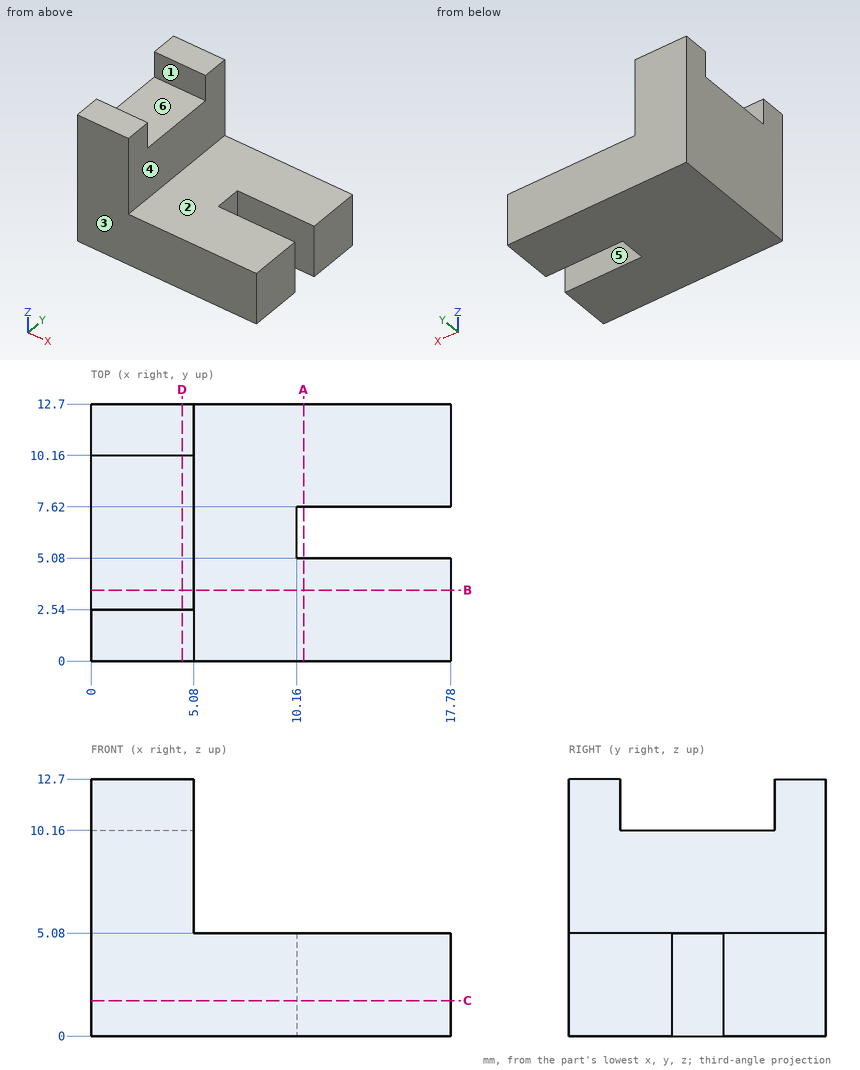
Answer from the drawing. Dimensions are ordinates in mm from the lowest x, y and z of the part. A direction names the side the tool comes from. Coordinates: 2 decimals unless noted, no trailing zeros. Loops run counter-clockwise (first coordinate to the right, second up) from the corner with the lowest first, then second, coordinate; pieces in that order, holes last. Notation, with made-up numbers: (61.25, -38.5) -> (118.25, -38.5) arc R20 ccw to (118.25, -3.5) -> close; hole circle Ø11 at (20.5, 38.25). An arc over 180 degrees is marked (long way). Return JSON: item names as keys, results as strings.
Item 1: Find section D-D (x = 4.5). Determine the outline of the cut face in (y, z), plus the area to 3 significant figures.
Answers:
{"outline": "(0, 0) -> (12.7, 0) -> (12.7, 12.7) -> (10.16, 12.7) -> (10.16, 10.16) -> (2.54, 10.16) -> (2.54, 12.7) -> (0, 12.7) -> close", "area": "142 mm2"}
Item 2: For a pull along Y with two mould halves and no side action, classify the marked faces 1, 2 and 3 as +Y half, -Y half, draft (parallel to the pull), parting line (faces both ways), or undercut.
Answers:
{"face 1": "undercut", "face 2": "draft", "face 3": "-Y half"}
Item 3: Find the intervals of material crossed by probe 1 along Y at (x, z) = (11.5, 1.5); probe 2 along X at (y, z) = (2.25, 12.25); probe 3 along Z at (x, y) = (1, 7.75), in increasing order.
Answers:
{"probe 1": "y = 0 to 5.08, 7.62 to 12.7", "probe 2": "x = 0 to 5.08", "probe 3": "z = 0 to 10.16"}
Item 4: Flat-ended cylindrical pins translate along their axes: P1, Ø2, axis at y = 9.5, z = 9.5, coming from the +X side; P2, Ø2, axis at x = 15.5, y = 7.5, coming from the -Z side; P3, Ø1.3, axis at y = 6.5, z = 1.5, coming from the +X side; P4, Ø1.5, axis at x = 15, y = 2.5, coming from the +Z side. Find the tip coordinate at first contact, or state that the pin passes through.
Answers:
{"P1": "stops at x = 5.08", "P2": "stops at z = 0", "P3": "stops at x = 10.16", "P4": "stops at z = 5.08"}
Item 5: For the marked faces 4, 5 and 6, determine the directions among +Z, -Z, +X, -X, +Y, -Y from which every point of the face is accessible in a straight line to the end or side of a thin tool.
Answers:
{"face 4": "+Z, +X, +Y, -Y", "face 5": "+Z, -Z, +X", "face 6": "+Z, +X, -X"}
Item 6: Find section A-A (x = 10.5). Determine the outline of the cut face in (y, z).
Answers:
{"outline": "(0, 0) -> (5.08, 0) -> (5.08, 5.08) -> (0, 5.08) -> close; (7.62, 0) -> (12.7, 0) -> (12.7, 5.08) -> (7.62, 5.08) -> close"}
Item 7: Find section B-B (y = 3.5). Determine the outline of the cut face in (x, z), plus the area to 3 significant figures.
Answers:
{"outline": "(0, 0) -> (17.78, 0) -> (17.78, 5.08) -> (5.08, 5.08) -> (5.08, 10.16) -> (0, 10.16) -> close", "area": "116 mm2"}
Item 8: Find section C-C (z = 1.75). Determine the outline of the cut face in (x, y).
Answers:
{"outline": "(0, 0) -> (17.78, 0) -> (17.78, 5.08) -> (10.16, 5.08) -> (10.16, 7.62) -> (17.78, 7.62) -> (17.78, 12.7) -> (0, 12.7) -> close"}
